Autodesk Inventor part; units mm, degrees
ref_plane "YZ Plane" through (0, 0, 0) normal (1, 0, 0) x (0, 1, 0)
ref_plane "XZ Plane" through (0, 0, 0) normal (0, 1, 0) x (-1, 0, 0)
ref_plane "XY Plane" through (0, 0, 0) normal (0, 0, 1) x (1, 0, 0)
sketch "スケッチ1" plane through (0, 0, 0) normal (0, 0, 1) x (1, 0, 0)
  line L0 (25, 2.5) -> (25, -2.5)
  line L1 (25, -2.5) -> (-25, -2.5)
  line L2 (-25, -2.5) -> (-25, 2.5)
  line L3 (-25, 2.5) -> (25, 2.5)
  point P0 (0, 0)
  dimension "d6" = 50
  dimension "d11" = 2.5
  dimension "d12" = 25
  dimension "d17" = 5
extrude "押し出し2" add sketch "スケッチ1" along normal blind 58
sketch "スケッチ2" plane through (0, 0, 58) normal (0, 0, 1) x (1, 0, 0)
  line L0 (25, 2.5) -> (-25, 2.5)
  circle A0 centre (-20, 0) radius 1
  circle A1 centre (20, 0) radius 1
  point P0 (0, 0)
  dimension "d20" = 2
  dimension "d22" = 40
  dimension "d23" = 20
  dimension "d24" = 2.5
  dimension "d25" = 2.5
hole "穴1" at (-20, 0, 58) at (20, 0, 58) direction (0, 0, -1) diameter 1.6 end through all
sketch "スケッチ3" plane through (-25, 2.5, 0) normal (0, 1, 0) x (1, 0, 0)
  line L0 (50, 0) -> (0, 0)
  line L1 (0, 0) -> (0, -58)
  line L2 (50, -58) -> (0, -58)
  line L3 (50, 0) -> (50, -58)
  line L4 (8, -5) -> (8, -53)
  line L5 (8, -53) -> (42, -5)
  line L6 (42, -5) -> (42, -53)
  line L7 (42, -53) -> (8, -5)
  line L8 (8, -5) -> (42, -5)
  line L9 (42, -53) -> (8, -53)
  line L10 (8, -10.1902) -> (38.3236, -53)
  line L11 (42, -47.8098) -> (11.6764, -5)
  line L12 (38.3236, -5) -> (8, -47.8098)
  line L13 (11.6764, -53) -> (42, -10.1902)
  point P0 (25, 0)
  dimension "d35" = 5
  dimension "d36" = 5
  dimension "d37" = 8
  dimension "d38" = 8
  dimension "d39" = 6
  dimension "d40" = 6
extrude "押し出し3" cut sketch "スケッチ3" against normal blind 5 contours L3 L2 L1 L0 | L7 L12 L10 L4 | L8 L11 L12 L7 | L12 L11 L5 L7 | L7 L5 L10 L12 | L12 L10 L5 L4 | L7 L13 L10 L5 | L5 L11 L13 L7 | L12 L8 L5 L11 | L5 L10 L13 L9 | L5 L6 L13 L11 | L13 L11 L6 L7 | L7 L9 L10 L13 keep common part
fillet "フィレット1" radius 1 12 edges at (-13.3236, 0, 5) (-17, 0, 10.1902) (0, 0, 23.8098) (-17, 0, 47.8098) (-3.6764, 0, 29) (13.3236, 0, 5) (0, 0, 34.1902) (17, 0, 10.1902) (17, 0, 47.8098) (13.3236, 0, 53) (-13.3236, 0, 53) (3.6764, 0, 29)
properties part number "Link_Supporter"
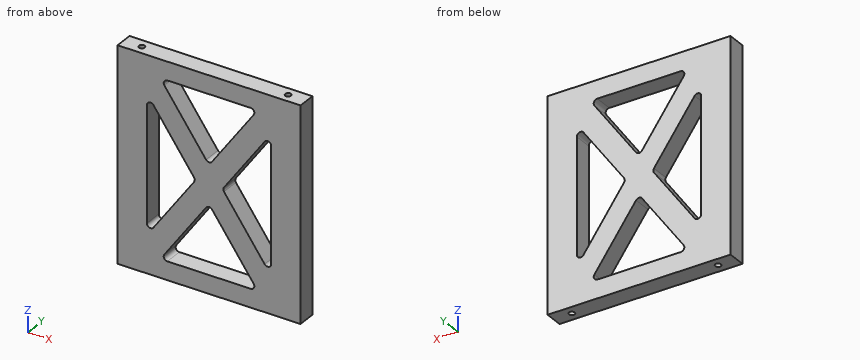
The model under review builds one solid part; all positions refer to its coordinate system, in mm. Give positions to 0.01 mm unless a question says otherwise; leave off trailing zeros. Loops run counter-clockwise (first coordinate to the right, second up) from the corner with the lowest first, then second, coordinate; pieces in that order, holes last. Notation, with made-up numbers: (-18.75, 34.5) -> (36.25, 34.5) arc R21 cw to (36.25, 61.5) -> close; hole circle Ø6 at (37, -35). An arc over 180 degrees is marked (long way). Answer as a JSON object with one key per item and string values. Group by question number.
Q1. Take a section at C-C (y = 0). State how many separate pieces and enclosed holes the cut face has, plus the area to 3 significant figures.
Q2. Take a section at D-D (z = 18). Write out the cut boundary in (x, y).
Q3. Take a section at B-B (x = -20). Write out the cut boundary in (y, z).
Q4. Take a section at A-A (z = 32). Write out the cut boundary in (x, y).
Q5. Insertion check: pin 1 (2 mm diameter, centred on x = -5.5, z = 29.5, fed in from +Y). The pin has a flat end and moves straight along its axis. Give the tip position at first contact, or say it passes through.
Q6. Wall thickness on line 1 along Z through (x, y) = (10.5, -0.35); line 2 along X through (y, z) = (1.6, 25.5); line 3 along X through (y, z) = (2.1, 26): over which ranges is each line inside the solid? List them lowest first.
Answer below:
{
 "1": {"separate pieces": "3", "enclosed holes": "4", "area": "1,720 mm2"},
 "2": {"outline": "(-25, -2.5) -> (-17, -2.5) -> (-17, 2.5) -> (-25, 2.5) -> close; (-11.47, -2.5) -> (-4.12, -2.5) -> (-4.12, 2.5) -> (-11.47, 2.5) -> close; (4.12, -2.5) -> (11.47, -2.5) -> (11.47, 2.5) -> (4.12, 2.5) -> close; (17, -2.5) -> (25, -2.5) -> (25, 2.5) -> (17, 2.5) -> close; hole circle Ø1.6 at (-20, 0); hole circle Ø1.6 at (20, 0)"},
 "3": {"outline": "(-2.5, 0) -> (-0.8, 0) -> (-0.8, 58) -> (-2.5, 58) -> close; (0.8, 0) -> (2.5, 0) -> (2.5, 58) -> (0.8, 58) -> close"},
 "4": {"outline": "(-25, -2.5) -> (-17, -2.5) -> (-17, 2.5) -> (-25, 2.5) -> close; (-5.8, -2.5) -> (5.8, -2.5) -> (5.8, 2.5) -> (-5.8, 2.5) -> close; (17, -2.5) -> (25, -2.5) -> (25, 2.5) -> (17, 2.5) -> close; hole circle Ø1.6 at (-20, 0); hole circle Ø1.6 at (20, 0)"},
 "5": {"pin 1": "passes through"},
 "6": {"line 1": "z = 0 to 5, 8.99 to 19.37, 38.63 to 49.01, 53 to 58", "line 2": "x = -25 to -17, -6.16 to 6.16, 17 to 25", "line 3": "x = -25 to -17, -5.8 to 5.8, 17 to 25"}
}
